The model under review builds one solid part; all positions refer to its coordinate system, in mm. Face numbers are marked on the shaded views. Coordinates: 2 decimals unless noted, no trailing zeros. Order: outer loops, then holes, each group sorted by start corner. A loop starts at its lowest first (then second) coordinate and runs counter-clockwise, first axis right, second up. Notation, with made-up numbers: (-34, 50.25) -> (-13, 50.25) arc R9 cw to (-13, 55.25) -> close; hole circle Ø1 at (-8.5, 35). An arc over 180 degrees is marked (long way). Use one line per item in the form item = value.
from build123d import *

# Parameters (mm, degrees)
F0_R     = 12.5
F0_R_2   = 3
F1_DEPTH = 10
F2_R     = 12.5
F2_R_2   = 3
F3_DEPTH = 2
F4_R     = 4.1082069006
F5_DEPTH = 3
F6_R     = 2.99999
F8_R     = 1
F9_SIZE  = 1


# Not quite as in the source:
# - a fillet or chamfer that OpenCascade refuses, or shapes differently, is made with other operations: its cross-section is extruded or revolved along the edge and cut away or added
# - a fillet or chamfer is up to 0.001 mm smaller than in the source, because OpenCascade refuses the exact size


with BuildPart() as f1:
    # F0 (on Top) → F1 (new body)
    with BuildSketch(Plane.XY):
        Circle(F0_R)
        Circle(F0_R_2, mode=Mode.SUBTRACT)
    extrude(amount=F1_DEPTH)

    # F2 (on face) → F3 (join)
    with BuildSketch(Plane.XY.offset(10)):
        Circle(F2_R)
        Circle(F2_R_2, mode=Mode.SUBTRACT)
        Circle(F2_R_2)
    extrude(amount=F3_DEPTH)

    # F4 (on face) → F5 (cut)
    with BuildSketch(Plane.XY.offset(12)):
        with Locations((-7.4370889924, 0)):
            Circle(F4_R)
    extrude(amount=-F5_DEPTH, mode=Mode.SUBTRACT)

    # F6 (radius 3 in the source; OpenCascade refuses exactly that, so slightly less here)
    f6_edges = [f1.edges().sort_by_distance(p)[0] for p in [
        (-11.545296, 0, 9),
    ]]
    fillet(f6_edges, radius=F6_R)

    # F7: fillet of radius 1 on 2 edges, made by hand

    # F7_s1 → F7_t2 (revolve, cut)
    with BuildSketch(Plane.XZ):
        with BuildLine():
            ThreePointArc((11.5, 12), (12.2071067812, 11.7071067812), (12.5, 11))
            Line((12.5, 11), (12.5, 12))
            Line((12.5, 12), (11.5, 12))
        make_face()
    revolve(axis=Axis((0, 0, 12), (0, 0, 1)), mode=Mode.SUBTRACT)

    # F7_s3 → F7_t4 (revolve, cut)
    with BuildSketch(Plane.XZ):
        with BuildLine():
            ThreePointArc((-3.4241428123, 11.249998125), (-3.0682696928, 11.7905688221), (-2.4558964916, 12))
            Line((-2.4558964916, 12), (-2.4558964916, 12.1))
            Line((-2.4558964916, 12.1), (-3.3288820918, 12.1))
            Line((-3.3288820918, 12.1), (-3.4288820918, 12))
            ThreePointArc((-3.4288820918, 12), (-3.4288820918, 11.99999), (-3.5209674443, 11.2749979375))
            Line((-3.5209674443, 11.2749979375), (-3.4241428123, 11.249998125))
        make_face()
    revolve(axis=Axis((-7.4370889924, 0, 12), (0, 0, 1)), mode=Mode.SUBTRACT)

    # F8
    f8_edges = [f1.edges().sort_by_distance(p)[0] for p in [
        (-12.5, 0, 0),
    ]]
    fillet(f8_edges, radius=F8_R)

    # F9
    f9_edges = [f1.edges().sort_by_distance(p)[0] for p in [
        (-3, 0, 0),
    ]]
    chamfer(f9_edges, length=F9_SIZE)


solid = f1.part
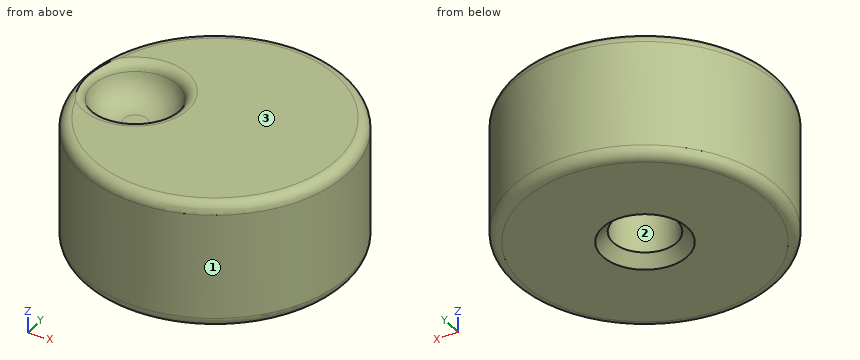
Item 1: To check wall thickness, follow L1, parallel to Y at x = 0, z = 5.25; L2, parallel to X at y = 5.5, z = 6.75; L3, parallel to Z at x = -10.25, y = 0.5. State the ranges of each line that lie inside material, in increasing order. Write a range as from..to.
Results found:
L1 = -12.5..-3, 3..12.5
L2 = -11.22..11.22
L3 = 0..9.56
Item 2: We need section A-A (x = 0). Write out the cut boundary in (y, z).
Results found:
outline = (-12.5, 1) arc R1 ccw to (-11.5, 0) -> (-4, 0) -> (-3, 1) -> (-3, 10) -> (3, 10) -> (3, 1) -> (4, 0) -> (11.5, 0) arc R1 ccw to (12.5, 1) -> (12.5, 11) arc R1 ccw to (11.5, 12) -> (-11.5, 12) arc R1 ccw to (-12.5, 11) -> close
Item 3: Draft analysis for pull direction Y (two halves, no side actions). For the marked faces 1, 2 and 3, state which applies: released by +Y, released by -Y, zero draft, split by the parting line, or undercut.
Results found:
face_1 = split by the parting line
face_2 = undercut
face_3 = zero draft
Item 4: We need section B-B (z = 7). Write out the cut boundary in (x, y), plus the area to 3 significant figures.
Results found:
outline = circle Ø25 at (0, 0); hole circle Ø6 at (0, 0)
area = 463 mm²
Item 5: Clearance check with flat-ended pins moving along their axes: pin 1 (2 mm diameter, centred on y = 8.5, z = 4.5, fed in from +X); pin 2 (5 mm diameter, centred on x = 0, y = 0, fed in from -Z); pin 3 (3 mm diameter, centred on y = 8, z = 7, fed in from +X). State where each tip first meets the part, or that it passes through.
Results found:
pin_1 = 10
pin_2 = 10
pin_3 = 10.68
